from build123d import *

# Parameters (mm, degrees)
ESQUISSE1_W              = 35
ESQUISSE1_H              = 25
BOSS_EXTRU_1_DEPTH       = 3
CONG_3_R                 = 7.5
ENL_V_MAT_EXTRU_2_REACH  = 45.116
ESQUISSE3_W              = 8
ESQUISSE3_H              = 3
ENL_V_MAT_EXTRU_3_REACH  = 45.116
ESQUISSE4_W              = 5.5
ESQUISSE4_H              = 3
ENL_V_START              = -3
ESQUISSE5_W              = 3.5
ESQUISSE5_H              = 11
ENL_V_MAT_EXTRU_4_DEPTH  = 3
ENL_V_MAT_EXTRU_7_REACH  = 45.116
ESQUISSE8_W              = 5
ESQUISSE8_H              = 3
ENL_V_MAT_EXTRU_8_REACH  = 45.116
ESQUISSE9_W              = 5
ESQUISSE9_H              = 3
ESQUISSE12_R             = 3
BOSS_EXTRU_2_DEPTH       = 2
ESQUISSE13_R             = 3
BOSS_EXTRU_4_DEPTH       = 2
ENL_V_MAT_EXTRU_11_REACH = 45.301
ESQUISSE14_R             = 1.25
ENL_V_MAT_EXTRU_12_REACH = 45.301
ESQUISSE15_R             = 1.25


with BuildPart() as part:
    # Esquisse1 → Boss.-Extru.1 (new body)
    with BuildSketch(Plane.XY):
        with Locations((17.5, 12.5)):
            Rectangle(ESQUISSE1_W, ESQUISSE1_H)
    extrude(amount=BOSS_EXTRU_1_DEPTH)

    # Congé3
    cong_3_edges = [part.edges().sort_by_distance(p)[0] for p in [
        (0, 25, 1.5),
        (35, 25, 1.5),
    ]]
    fillet(cong_3_edges, radius=CONG_3_R)

    # Esquisse3 → Enlèv. mat.-Extru.2 (cut, up to next)
    with BuildSketch(Plane.XY.offset(3), mode=Mode.PRIVATE) as enl_v_mat_extru_2_sk1:
        with Locations((17.5, 1.5)):
            Rectangle(ESQUISSE3_W, ESQUISSE3_H)
    enl_v_mat_extru_2_tool1 = extrude(enl_v_mat_extru_2_sk1.sketch, amount=-ENL_V_MAT_EXTRU_2_REACH, mode=Mode.PRIVATE) & part.part
    add(enl_v_mat_extru_2_tool1.solids().sort_by_distance((17.5, 1.5, 3))[0], mode=Mode.SUBTRACT)

    # Esquisse4 → Enlèv. mat.-Extru.3 (cut, up to next)
    with BuildSketch(Plane.XY.offset(3), mode=Mode.PRIVATE) as enl_v_mat_extru_3_sk1:
        with Locations((17.5, 7.5)):
            Rectangle(ESQUISSE4_W, ESQUISSE4_H)
    enl_v_mat_extru_3_tool1 = extrude(enl_v_mat_extru_3_sk1.sketch, amount=-ENL_V_MAT_EXTRU_3_REACH, mode=Mode.PRIVATE) & part.part
    add(enl_v_mat_extru_3_tool1.solids().sort_by_distance((17.5, 7.5, 3))[0], mode=Mode.SUBTRACT)

    # Esquisse5 → Enlèv. mat.-Extru.4 (cut)
    with BuildSketch(Plane.XY.offset(3).offset(ENL_V_START)):
        with Locations((17.5, 5.5)):
            Rectangle(ESQUISSE5_W, ESQUISSE5_H)
    extrude(amount=ENL_V_MAT_EXTRU_4_DEPTH, mode=Mode.SUBTRACT)

    # Esquisse8 → Enlèv. mat.-Extru.7 (cut, up to next)
    with BuildSketch(Plane.XY.offset(3), mode=Mode.PRIVATE) as enl_v_mat_extru_7_sk1:
        with Locations((2.5, 1.5)):
            Rectangle(ESQUISSE8_W, ESQUISSE8_H)
    enl_v_mat_extru_7_tool1 = extrude(enl_v_mat_extru_7_sk1.sketch, amount=-ENL_V_MAT_EXTRU_7_REACH, mode=Mode.PRIVATE) & part.part
    add(enl_v_mat_extru_7_tool1.solids().sort_by_distance((2.5, 1.5, 3))[0], mode=Mode.SUBTRACT)

    # Esquisse9 → Enlèv. mat.-Extru.8 (cut, up to next)
    with BuildSketch(Plane.XY.offset(3), mode=Mode.PRIVATE) as enl_v_mat_extru_8_sk1:
        with Locations((32.5, 1.5)):
            Rectangle(ESQUISSE9_W, ESQUISSE9_H)
    enl_v_mat_extru_8_tool1 = extrude(enl_v_mat_extru_8_sk1.sketch, amount=-ENL_V_MAT_EXTRU_8_REACH, mode=Mode.PRIVATE) & part.part
    add(enl_v_mat_extru_8_tool1.solids().sort_by_distance((32.5, 1.5, 3))[0], mode=Mode.SUBTRACT)

    # Esquisse12 → Boss.-Extru.2 (add)
    with BuildSketch(Plane.XY.offset(3)):
        with Locations(Location((30, 19, 0), (0, 0, 180))):
            Circle(ESQUISSE12_R)
    extrude(amount=BOSS_EXTRU_2_DEPTH)

    # Esquisse13 → Boss.-Extru.4 (add)
    with BuildSketch(Plane.XY.offset(3)):
        with Locations(Location((5, 19, 0), (0, 0, 180))):
            Circle(ESQUISSE13_R)
    extrude(amount=BOSS_EXTRU_4_DEPTH)

    # Esquisse14 → Enlèv. mat.-Extru.11 (cut, up to next)
    with BuildSketch(Plane.XY.offset(5), mode=Mode.PRIVATE) as enl_v_mat_extru_11_sk1:
        with Locations((5, 19)):
            Circle(ESQUISSE14_R)
    enl_v_mat_extru_11_tool1 = extrude(enl_v_mat_extru_11_sk1.sketch, amount=-ENL_V_MAT_EXTRU_11_REACH, mode=Mode.PRIVATE) & part.part
    add(enl_v_mat_extru_11_tool1.solids().sort_by_distance((5, 19, 5))[0], mode=Mode.SUBTRACT)

    # Esquisse15 → Enlèv. mat.-Extru.12 (cut, up to next)
    with BuildSketch(Plane.XY.offset(5), mode=Mode.PRIVATE) as enl_v_mat_extru_12_sk1:
        with Locations((30, 19)):
            Circle(ESQUISSE15_R)
    enl_v_mat_extru_12_tool1 = extrude(enl_v_mat_extru_12_sk1.sketch, amount=-ENL_V_MAT_EXTRU_12_REACH, mode=Mode.PRIVATE) & part.part
    add(enl_v_mat_extru_12_tool1.solids().sort_by_distance((30, 19, 5))[0], mode=Mode.SUBTRACT)


solid = part.part
The listing builds one solid part. Answer for the finished solid, in the listing's coordinates (mm). A direction names the side the tool comes from. Coordinates: 2 decimals unless noted, no trailing zeros. Order: outer loops, then holes, each group sorted by start corner. A loop starts at its lowest first (then second) coordinate and runs counter-clockwise, first axis right, second up. Notation, with made-up numbers: (70, -4) -> (94, -4) arc R10 ccw to (94, 7) -> close; hole circle Ø5 at (-10.75, -19). An arc over 180 degrees is marked (long way). Answer in a Markdown table with one row per item. Add a question column.
Item 1: Which of the six approach directions +Z, -Z, +X, -X, +Y, -Y give full straight-line access (tool end or side, diameter ignored) to faces 1 (the face through (15, 6, 2)), 2 (the face through (5, 1, 2)), 3 (the face through (15, 3, 2))?
Item 2: Each of these flat-tipped pins is pushed along its axis until it touches: P1, Ø10, axis at x = 14, y = 10, coming from the -Z side; P2, Ø2, axis at y = 22, z = 2, coming from the +X side; P3, Ø1.5, axis at y = 1, z = 1, coming from the +X side; P4, Ø2.5, axis at y = 1, z = 2, coming from the -X side. Where does it stop, or does it pass through?
Item 3: Find the intervals of material crossed by L1, parallel to X at y = 1.5, z = 1.85; L2, parallel to X at y = 19.5, z = 3.9; L3, parallel to Y at x = 30, z = 3.95, in increasing order. Write a range as from..to.
Item 4: Find section A-A (y = 2.5). Write down the section's boundary in (x, z), then the cut area to 3 significant figures.
Item 5: Find section B-B (z = 4). Write down the section's boundary in (x, y), then the cut area to 3 significant figures.
Item 6: Determine the mould class of faces 4 (the face through (17, 11, 1)), 5 (the face through (2, 3, 2)), 6 (the face through (32.861, 22.745, 1.521)) for opening direction X: +X half, -X half, draft (parallel to the pull), parting line (faces both ways), or undercut.
Item 7: Find section C-C (y = 7.5). Write down the section's boundary in (x, z).
Item 8: Find section D-D (z = 0.9). Write down the section's boundary in (x, y), then the cut area to 3 significant figures.
Result set:
| question | item | result |
|---|---|---|
| 1 | face 1 | +Z, -Z |
| 1 | face 2 | +Z, -Z, -X, -Y |
| 1 | face 3 | +Z, -Z, -Y |
| 2 | P1 | stops at z = 0 |
| 2 | P2 | stops at x = 34.13 |
| 2 | P3 | stops at x = 30 |
| 2 | P4 | stops at x = 5 |
| 3 | L1 | x = 5..13.5, 21.5..30 |
| 3 | L2 | x = 2.04..3.85, 6.15..7.96, 27.04..28.85, 31.15..32.96 |
| 3 | L3 | y = 16..17.75, 20.25..22 |
| 4 | outline | (5, 0) -> (13.5, 0) -> (13.5, 3) -> (5, 3) -> close; (21.5, 0) -> (30, 0) -> (30, 3) -> (21.5, 3) -> close |
| 4 | area | 51.0 mm² |
| 5 | outline | circle Ø6 at (5, 19); circle Ø6 at (30, 19); hole circle Ø2.5 at (5, 19); hole circle Ø2.5 at (30, 19) |
| 5 | area | 46.7 mm² |
| 6 | face 4 | undercut |
| 6 | face 5 | draft |
| 6 | face 6 | +X half |
| 7 | outline | (0, 0) -> (14.75, 0) -> (14.75, 3) -> (0, 3) -> close; (20.25, 0) -> (35, 0) -> (35, 3) -> (20.25, 3) -> close |
| 8 | outline | (0, 3) -> (5, 3) -> (5, 0) -> (13.5, 0) -> (13.5, 3) -> (15.75, 3) -> (15.75, 6) -> (14.75, 6) -> (14.75, 9) -> (15.75, 9) -> (15.75, 11) -> (19.25, 11) -> (19.25, 9) -> (20.25, 9) -> (20.25, 6) -> (19.25, 6) -> (19.25, 3) -> (21.5, 3) -> (21.5, 0) -> (30, 0) -> (30, 3) -> (35, 3) -> (35, 17.5) arc R7.5 ccw to (27.5, 25) -> (7.5, 25) arc R7.5 ccw to (0, 17.5) -> close; hole circle Ø2.5 at (5, 19); hole circle Ø2.5 at (30, 19) |
| 8 | area | 753 mm² |
